Autodesk Inventor part; units mm, degrees
ref_plane "YZ Plane" through (0, 0, 0) normal (1, 0, 0) x (0, 1, 0)
ref_plane "XZ Plane" through (0, 0, 0) normal (0, 1, 0) x (-1, 0, 0)
ref_plane "XY Plane" through (0, 0, 0) normal (0, 0, 1) x (1, 0, 0)
sketch "Sketch1" plane through (0, 0, 0) normal (1, 0, 0) x (0, 1, 0)
  arc A0 (30.9, 0) -> (12.381, 28.3112) centre (0, 0) ccw
  arc A1 (44.1, 0) -> (17.6699, 40.4052) centre (0, 0) ccw
  line L0 (12.381, 28.3112) -> (17.6699, 40.4052)
  line L1 (30.9, 0) -> (44.1, 0) construction
  arc A2 (17.6699, 40.4052) -> (12.381, 28.3112) centre (15.0255, 34.3582) ccw
  arc A3 (30.9, 0) -> (44.1, 0) centre (37.5, 0) ccw
  circle A4 centre (15.0255, 34.3582) radius 2.1
  circle A5 centre (37.5, 0) radius 2.1
  dimension "d0" = 61.8
  dimension "d1" = 88.2
  dimension "d2" = 66.379
  dimension "d3" = 4.2
  dimension "d4" = 4.2
extrude "Extrusion1" add sketch "Sketch1" along normal blind 3 contours A0 L0 A4 A1 A3 | A2 L0 A4
chamfer "Chamfer1" distance 2.15 distance2 3 2 edges at (3, 12.9255, 34.3582) (3, 35.4, 0) measured on face at (3, 38.069, 10.7229)
properties part number "Mechanische_Anschlaege_Clip"
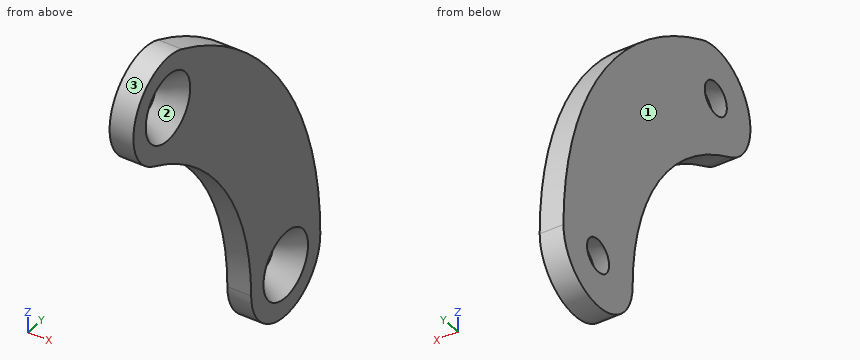
Read the model definition and answer for the solid it produces. Units are mm, in the model's axes. Face numbers are marked on the shaded views. Give positions to 0.01 mm unless a question says otherwise; leave off trailing zeros. Write each loop counter-clockwise with the first axis right and the second up, starting at its lowest first coordinate (ties: lowest second). Pieces come first, ordered by that corner, then holes. Notation, with made-up numbers: (-18, 26.5) - (9, 26.5) arc R10 cw to (9, 39.5) - close; hole circle Ø4 at (-26, -38). An arc over 180 degrees is marked (long way). Write item = value, one per line. Start each with the question number.
Item 1: Find section C-C (z = 22). Give the vertices of the cut face in (x, y), then the cut area to 3 significant figures.
Item 2: Find section B-B (x = 0.75). Give the vertices of the cut face in (y, z), then the cut area to 3 significant figures.
Item 3: Each of these flat-tipped pins is pushed along its axis until it touches: P1, Ø5.5, axis at y = 37.5, z = 0, coming from the +X side; P2, Ø2, axis at y = 16, z = 26, coming from the -X side. Where does it stop, or does it pass through?
Item 4: The mould has two halves that part along Y. Classify the marked faces 1, 2 and 3: +Y half, -Y half, draft (parallel to the pull), parting line (faces both ways), or undercut.
Item 5: Find the intervals of material crossed by probe 1 along Z at (x, y) = (0.05, 37.5); probe 2 along Y at (x, z) = (1.05, 36.5); probe 3 along Z at (x, y) = (1.9, 12), in increasing order. Write a range as [from, to].
Item 6: Find section D-D (y = 32). Give the vertices of the cut face in (x, z), then the cut area to 3 significant figures.
Response:
q1.outline = (0, 21.7) - (3, 21.7) - (3, 38.22) - (0, 38.22) - close
q1.area = 49.6 mm²
q2.outline = (12.38, 28.31) arc R30.9 cw to (30.9, 0) arc R6.6 ccw to (44.1, 0) arc R44.1 ccw to (17.67, 40.41) arc R6.6 ccw to start; hole circle Ø5.27 at (15.03, 34.36); hole circle Ø5.27 at (37.5, 0)
q2.area = 667 mm²
q3.P1 = 0.91
q3.P2 = 0
q4.face_1 = draft
q4.face_2 = undercut
q4.face_3 = parting line
q5.probe_1 = [-6.6, -2.14], [2.14, 23.21]
q5.probe_2 = [8.78, 13.14], [16.91, 24.75]
q5.probe_3 = [28.49, 32.68], [36.04, 40.22]
q6.outline = (0, -3.65) - (3, -3.65) - (3, 30.34) - (0, 30.34) - close
q6.area = 102 mm²
